from build123d import *

# Parameters (mm, degrees)
BOSS_EXTRUDE3_DEPTH             = 127.2
CUT_EXTRUDE1_DEPTH              = 128.798043803
BOSS_EXTRUDE5_REACH             = 129.798
LPATTERN3_COUNT                 = 30
LPATTERN3_PITCH                 = 3.18
LPATTERN3_COL_COUNT             = 11
LPATTERN3_COL_PITCH             = 3.18
FILLET2_R                       = 1
SKETCH9_W                       = 28
SKETCH9_H                       = 4.5
BOSS_EXTRUDE6_DEPTH             = 8
BOSS_EXTRUDE6_DIRECTION_2_REACH = 129.798


with BuildPart() as part:
    # Sketch4 → Boss-Extrude3 (new body)
    with BuildSketch(Plane(origin=(0, 0, 0), x_dir=(0, 0, -1), z_dir=(1, 0, 0))):
        Polygon((0, 0), (-4.5, 0), (-4.5, 11.5), (-2.5, 11.5), (-2.5, 8), (0, 8), align=None)
    extrude(amount=BOSS_EXTRUDE3_DEPTH)

    # Sketch6 → Cut-Extrude1 (cut, through all)
    with BuildSketch(Plane.XY.offset(4.5)):
        with BuildLine():
            Line((87.45, 5.3), (119.25, 5.3))
            ThreePointArc((119.25, 5.3), (120.55, 4), (119.25, 2.7))
            Line((119.25, 2.7), (87.45, 2.7))
            ThreePointArc((87.45, 2.7), (86.15, 4), (87.45, 5.3))
        make_face()
    extrude(amount=-CUT_EXTRUDE1_DEPTH, mode=Mode.SUBTRACT)

    # Sketch8 → Boss-Extrude5 (add, up to next)
    with BuildSketch(Plane(origin=(0, 0, 0), x_dir=(-1, 0, 0), z_dir=(0, 0, -1)), mode=Mode.PRIVATE) as boss_extrude5_sk1:
        Polygon((-94.952664599, 8), (-94.327664599, 10), (-93.577664599, 10), (-92.952664599, 8), align=None)
    boss_extrude5_tool1 = extrude(boss_extrude5_sk1.sketch, amount=-BOSS_EXTRUDE5_REACH, mode=Mode.PRIVATE) - part.part
    boss_extrude5 = boss_extrude5_tool1.solids().sort_by_distance((93.952665, 8.848485, 0))[0]
    add(boss_extrude5)

    # LPattern3: Boss-Extrude5 ×30
    with Locations(*[(-i * LPATTERN3_PITCH, 0, 0) for i in range(1, LPATTERN3_COUNT)]):
        add(boss_extrude5)

    # LPattern3 col: Boss-Extrude5 ×11
    with Locations(*[(i * LPATTERN3_COL_PITCH, 0, 0) for i in range(1, LPATTERN3_COL_COUNT)]):
        add(boss_extrude5)

    # Fillet2
    fillet2_edges = [part.edges().sort_by_distance(p)[0] for p in [
        (63.6, 11.5, 2.5),
    ]]
    fillet(fillet2_edges, radius=FILLET2_R)

    # Sketch9 → Boss-Extrude6 (add)
    with BuildSketch(Plane(origin=(0, 11.5, 0), x_dir=(1, 0, 0), z_dir=(0, 1, 0))):
        with Locations((113.2, -2.25)):
            Rectangle(SKETCH9_W, SKETCH9_H)
    extrude(amount=BOSS_EXTRUDE6_DEPTH)

    # Sketch9 → Boss-Extrude6 direction 2 (add, up to next)
    with BuildSketch(Plane(origin=(0, 11.5, 0), x_dir=(1, 0, 0), z_dir=(0, 1, 0)), mode=Mode.PRIVATE) as boss_extrude6_direction_2_sk1:
        with Locations((113.2, -2.25)):
            Rectangle(SKETCH9_W, SKETCH9_H)
    boss_extrude6_direction_2_tool1 = extrude(boss_extrude6_direction_2_sk1.sketch, amount=-BOSS_EXTRUDE6_DIRECTION_2_REACH, mode=Mode.PRIVATE) - part.part
    add(boss_extrude6_direction_2_tool1.solids().sort_by_distance((113.2, 11.5, 2.25))[0])


solid = part.part
The model under review builds one solid part; all positions refer to its coordinate system, in mm. A direction names the side the tool comes from. Coordinates: 2 decimals unless noted, no trailing zeros. Write each loop counter-clockwise with the first axis right and the second up, starting at its lowest first coordinate (ties: lowest second). Pieces come first, ordered by that corner, then holes. Notation, with made-up numbers: (83.25, -15) -> (101.25, -15) arc R19 ccw to (101.25, 9) -> close; hole circle Ø2 at (75.25, 86.25). An arc over 180 degrees is marked (long way). Answer in a Markdown table with one row per item.
1. We need section A-A, the plane y = 4. State the section outline as (x, z) points, and give its area (3 significant figures).
Answers below:
| item | result |
|---|---|
| outline | (0, 0) -> (86.15, 0) -> (86.15, 4.5) -> (0, 4.5) -> close; (120.55, 0) -> (127.2, 0) -> (127.2, 4.5) -> (120.55, 4.5) -> close |
| area | 418 mm^2 |
2. For faces 3 (the cylindrical face through (120.55, 4.03, 2.28)), 4 (the flat face through (76.8, 7.7, 0)), 5 (the flat face through (42.39, 9.01, 1.23)), list the 3-axis set-ups (+Z, -Z, +X, -X, +Y, -Y) from which the entire face can be reached by the end or side of a thin tool; tool diameter is ignored.
Answers below:
| item | result |
|---|---|
| face 3 | +Z, -Z |
| face 4 | -Z, +X, -X, +Y, -Y |
| face 5 | -Z, +Y |
3. Draft analysis for pull direction X (two halves, no side actions). For faces 1 (the flat face through (64.65, 9.01, 1.23)), 2 (the flat face through (63, 7, 4.5)), state which applies: +X half, -X half, draft (parallel to the pull), parting line (faces both ways), or undercut.
Answers below:
| item | result |
|---|---|
| face 1 | undercut |
| face 2 | draft |
4. Clearance check with flat-ended pins moving along their axes: pin 1 Ø0.8 at (x, z) = (5, 1) entering from +Y; pin 2 Ø0.5 at (x, z) = (46.5, 4) entering from +Y; pin 3 Ø0.6 at (x, z) = (86, 1.5) entering from +Y. State where each tip first meets the part, or that it passes through.
Answers below:
| item | result |
|---|---|
| pin 1 | stops at y = 10 |
| pin 2 | stops at y = 11.5 |
| pin 3 | stops at y = 8 |
5. We need section B-B, the plane y = 13.25. State the section outline as (x, z) points.
Answers below:
| item | result |
|---|---|
| outline | (99.2, 0) -> (127.2, 0) -> (127.2, 4.5) -> (99.2, 4.5) -> close |
6. Wall thickness on probe 1 along Y at (x, z) = (113, 2.7); probe 2 along X at (y, z) = (13.25, 3.85); probe 3 along Y at (x, z) = (35.5, 1.25): over which ranges is each line inside the solid? List them lowest first. Write a range as [from, to].
Answers below:
| item | result |
|---|---|
| probe 1 | y = [0, 2.7], [5.3, 19.5] |
| probe 2 | x = [99.2, 127.2] |
| probe 3 | y = [0, 8] |
